Input: dimensioned drawing with shaded views. Units: mm. Origin: part minimum x, y, z. A direction names the side the tool comes from. Give positions to 0.01 mm unless a question says otherwise; leave off trailing zeros. Loops run counter-clockwise (first coordinate to the right, second up) from the corner with the lowest first, then second, coordinate; pieces in that order, holes last.
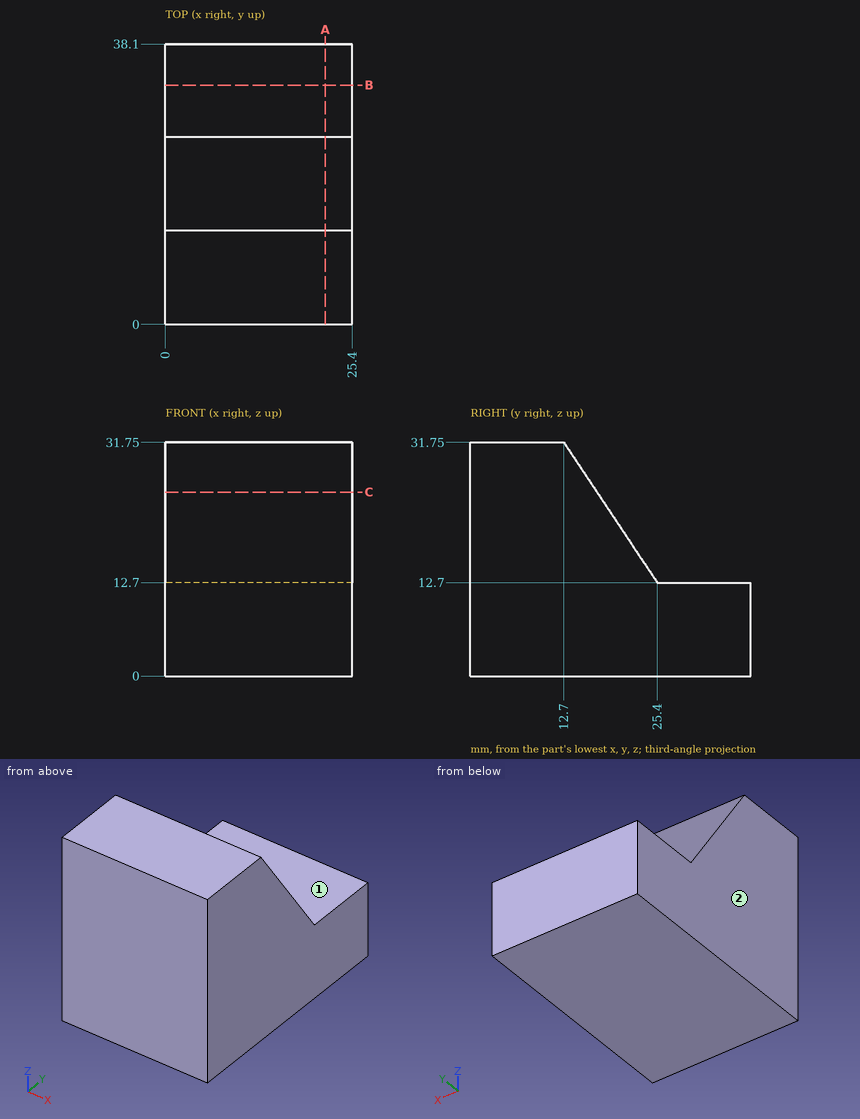
(1) Reachability of the marked faces 1 and 2 from +Z, -Z, +X, -X, +Y, -Y: full face, straight path, thin tool, end or side. Return the list, or none.
A:
face 1: +Z, +X, -X, +Y
face 2: +Z, -Z, -X, +Y, -Y
(2) Section C-C, the plane z = 25. Return the cut outline in (x, y).
A:
outline: (0, 0) - (25.4, 0) - (25.4, 17.2) - (0, 17.2) - close
(3) First-contact query: pin 1 (4 mm diameter, centred on x = 19.5, y = 10.5, fed in from -Z); pin 2 (6.5 mm diameter, centred on x = 9, y = 30, fed in from +Z). Flat tips, straight axial feed; report the tip coordinate or a pass-through.
A:
pin 1: stops at z = 0
pin 2: stops at z = 12.7
(4) Ray query, line 1 along Z through (x, y) = (8.25, 30.5); line 2 along Y through (x, z) = (12, 24); line 3 along Y through (x, z) = (18.5, 18). Return the intervals inside material, ascending.
A:
line 1: z = 0 to 12.7
line 2: y = 0 to 17.87
line 3: y = 0 to 21.87
(5) Section B-B, the plane y = 32.5. Return the cut outline in (x, z).
A:
outline: (0, 0) - (25.4, 0) - (25.4, 12.7) - (0, 12.7) - close
(6) Section A-A, the plane x = 21.75. Return the cut outline in (y, z), then the cut area to 3 significant figures.
A:
outline: (0, 0) - (38.1, 0) - (38.1, 12.7) - (25.4, 12.7) - (12.7, 31.75) - (0, 31.75) - close
area: 847 mm2
